Design review of the part built by this model. Coordinates are the model's own, in mm. A direction names the side the tool comes from. Give positions to 0.01 mm unless a question says otherwise; leave off trailing zeros. Order: outer loops, then holes, each group sorted by start corner. A loop starts at its lowest first (then second) coordinate and runs counter-clockwise, first axis right, second up.
```python
from build123d import *

# Parameters (mm, degrees)
SKETCH_1_R          = 1.55
SKETCH_1_W          = 30.4
SKETCH_1_H          = 68.58
EXTRUDE_1_DEPTH     = 1.5
FILLET_1_R          = 10
FILLET_2_R          = 10
FILLET_3_R          = 10
SKETCH_1_5_R        = 2
CUT_EXTRUDE_3_DEPTH = 10


with BuildPart() as part:
    # 草图1 → 凸台-拉伸1 (new body)
    with BuildSketch(Plane(origin=(0, 0, 0), x_dir=(1, 0, 0), z_dir=(0, 1, 0))):
        with BuildLine():
            Line((-125, 175), (-175, 125))
            Line((-175, 125), (-175, -125))
            Line((-175, -125), (-125, -175))
            Line((-125, -175), (-81.710313025, -175))
            ThreePointArc((-81.710313025, -175), (0, -122.728301649), (81.710313025, -175))
            Line((81.710313025, -175), (125, -175))
            Line((125, -175), (175, -125))
            Line((175, -125), (175, 125))
            Line((175, 125), (125, 175))
            Line((125, 175), (85, 175))
            Line((85, 175), (40, 125))
            Line((40, 125), (40, 85))
            Line((40, 85), (-40, 85))
            Line((-40, 85), (-40, 125))
            Line((-40, 125), (-85, 175))
            Line((-85, 175), (-125, 175))
        make_face()
        with Locations((-55, 131)):
            Circle(SKETCH_1_R, mode=Mode.SUBTRACT)
        with Locations((-80, 160)):
            Circle(SKETCH_1_R, mode=Mode.SUBTRACT)
        with Locations((55, 131)):
            Circle(SKETCH_1_R, mode=Mode.SUBTRACT)
        with Locations((80, 160)):
            Circle(SKETCH_1_R, mode=Mode.SUBTRACT)
        with Locations((-65, 118.58)):
            Circle(SKETCH_1_R, mode=Mode.SUBTRACT)
        with Locations((-65, 50)):
            Circle(SKETCH_1_R, mode=Mode.SUBTRACT)
        with Locations((-110.72, 50)):
            Circle(SKETCH_1_R, mode=Mode.SUBTRACT)
        with Locations((-110.72, 118.58)):
            Circle(SKETCH_1_R, mode=Mode.SUBTRACT)
        with Locations((-164.434, 118.58)):
            Circle(SKETCH_1_R, mode=Mode.SUBTRACT)
        with Locations((-164.434, 50)):
            Circle(SKETCH_1_R, mode=Mode.SUBTRACT)
        with Locations((-65, -118.58)):
            Circle(SKETCH_1_R, mode=Mode.SUBTRACT)
        with Locations((-65, -50)):
            Circle(SKETCH_1_R, mode=Mode.SUBTRACT)
        with Locations((-110.72, -50)):
            Circle(SKETCH_1_R, mode=Mode.SUBTRACT)
        with Locations((-110.72, -118.58)):
            Circle(SKETCH_1_R, mode=Mode.SUBTRACT)
        with Locations((-164.434, -50)):
            Circle(SKETCH_1_R, mode=Mode.SUBTRACT)
        with Locations((-164.434, -118.58)):
            Circle(SKETCH_1_R, mode=Mode.SUBTRACT)
        with Locations((65, 50)):
            Circle(SKETCH_1_R, mode=Mode.SUBTRACT)
        with Locations((110.72, 50)):
            Circle(SKETCH_1_R, mode=Mode.SUBTRACT)
        with Locations((110.72, 118.58)):
            Circle(SKETCH_1_R, mode=Mode.SUBTRACT)
        with Locations((65, 118.58)):
            Circle(SKETCH_1_R, mode=Mode.SUBTRACT)
        with Locations((164.434, 118.58)):
            Circle(SKETCH_1_R, mode=Mode.SUBTRACT)
        with Locations((164.434, 50)):
            Circle(SKETCH_1_R, mode=Mode.SUBTRACT)
        with Locations((164.434, -118.58)):
            Circle(SKETCH_1_R, mode=Mode.SUBTRACT)
        with Locations((164.434, -50)):
            Circle(SKETCH_1_R, mode=Mode.SUBTRACT)
        with Locations((110.72, -50)):
            Circle(SKETCH_1_R, mode=Mode.SUBTRACT)
        with Locations((110.72, -118.58)):
            Circle(SKETCH_1_R, mode=Mode.SUBTRACT)
        with Locations((65, -118.58)):
            Circle(SKETCH_1_R, mode=Mode.SUBTRACT)
        with Locations((65, -50)):
            Circle(SKETCH_1_R, mode=Mode.SUBTRACT)
        with Locations((-138.794, 84.29)):
            Rectangle(SKETCH_1_W, SKETCH_1_H, mode=Mode.SUBTRACT)
        with Locations((138.794, 84.29)):
            Rectangle(SKETCH_1_W, SKETCH_1_H, mode=Mode.SUBTRACT)
        with Locations((-138.794, -84.29)):
            Rectangle(SKETCH_1_W, SKETCH_1_H, mode=Mode.SUBTRACT)
        with Locations((138.794, -84.29)):
            Rectangle(SKETCH_1_W, SKETCH_1_H, mode=Mode.SUBTRACT)
    extrude(amount=EXTRUDE_1_DEPTH)

    # 圆角1
    fillet_1_edges = [part.edges().sort_by_distance(p)[0] for p in [
        (-40, 0.75, -125),
    ]]
    fillet(fillet_1_edges, radius=FILLET_1_R)

    # 圆角2
    fillet_2_edges = [part.edges().sort_by_distance(p)[0] for p in [
        (40, 0.75, -125),
    ]]
    fillet(fillet_2_edges, radius=FILLET_2_R)

    # 圆角3
    fillet_3_edges = [part.edges().sort_by_distance(p)[0] for p in [
        (175, 0.75, 125),
        (125, 0.75, 175),
        (81.710313025, 0.75, 175),
        (-81.710313025, 0.75, 175),
        (-125, 0.75, 175),
        (-175, 0.75, 125),
        (-175, 0.75, -125),
        (-125, 0.75, -175),
        (-85, 0.75, -175),
        (85, 0.75, -175),
        (125, 0.75, -175),
        (175, 0.75, -125),
    ]]
    fillet(fillet_3_edges, radius=FILLET_3_R)

    # 草图1<5> → 切除-拉伸3 (cut)
    with BuildSketch(Plane(origin=(0, 0, 0), x_dir=(1, 0, 0), z_dir=(0, 1, 0))):
        with Locations((58.5, 118.58)):
            Circle(SKETCH_1_5_R)
        with Locations((43.5, 118.58)):
            Circle(SKETCH_1_5_R)
        with Locations((58.5, 108.58)):
            Circle(SKETCH_1_5_R)
        with Locations((43.5, 108.58)):
            Circle(SKETCH_1_5_R)
        with Locations((-43.5, 108.58)):
            Circle(SKETCH_1_5_R)
        with Locations((-58.5, 118.58)):
            Circle(SKETCH_1_5_R)
        with Locations((-58.5, 108.58)):
            Circle(SKETCH_1_5_R)
        with Locations((-43.5, 118.58)):
            Circle(SKETCH_1_5_R)
    extrude(amount=CUT_EXTRUDE_3_DEPTH, mode=Mode.SUBTRACT)


solid = part.part
```
1. Take a section at A-A (z = -70). State the section outline as (x, y) points.
Recorded:
outline: (-175, 0) - (-153.99, 0) - (-153.99, 1.5) - (-175, 1.5) - close; (-123.59, 0) - (123.59, 0) - (123.59, 1.5) - (-123.59, 1.5) - close; (153.99, 0) - (175, 0) - (175, 1.5) - (153.99, 1.5) - close
2. Take a section at C-C (x = 11). State the section outline as (y, z) points, then the cut area to 3 significant figures.
Recorded:
outline: (0, -85) - (1.5, -85) - (1.5, 123.4) - (0, 123.4) - close
area: 313 mm2
3. For line 1 along X through (y, z) = (1.3, -53); line 2 along X through (y, z) = (1.2, -104.5); line 3 along Z through (x, y) = (-111, 0.65), list the stretches that pass through material, from the lowest coordinate up.
Recorded:
line 1: x = -175 to -153.99, -123.59 to 123.59, 153.99 to 175
line 2: x = -175 to -153.99, -123.59 to -40, 40 to 123.59, 153.99 to 175
line 3: z = -175 to -120.1, -117.06 to -51.52, -48.48 to 48.48, 51.52 to 117.06, 120.1 to 175
4. Machinability: for faces 1 (the face through (-150, 1, 150)), 2 (the face through (62.57, 0.74, -150.08)), which of the approach directions +Z, -Z, +X, -X, +Y, -Y give a long, thin tool a straight path to every point of the face, cutting with its end or side? Answer none if there is none.
Recorded:
face 1: +Z, -X, +Y, -Y
face 2: -Z, +Y, -Y
5. Take a section at B-B (y = 0.6). State how many separate pieces and enclosed holes the cut face has, then the cut area to 3 significant figures.
Recorded:
separate pieces: 1
enclosed holes: 40
area: 93,200 mm2
6. For pin 1 (0.8 mm diameter, centred on x = 133.5, y = 1, fed in from +Z), flat-tipped, find the tip position at first contact; note if it passes through.
Recorded:
pin 1: stops at z = 166.9
